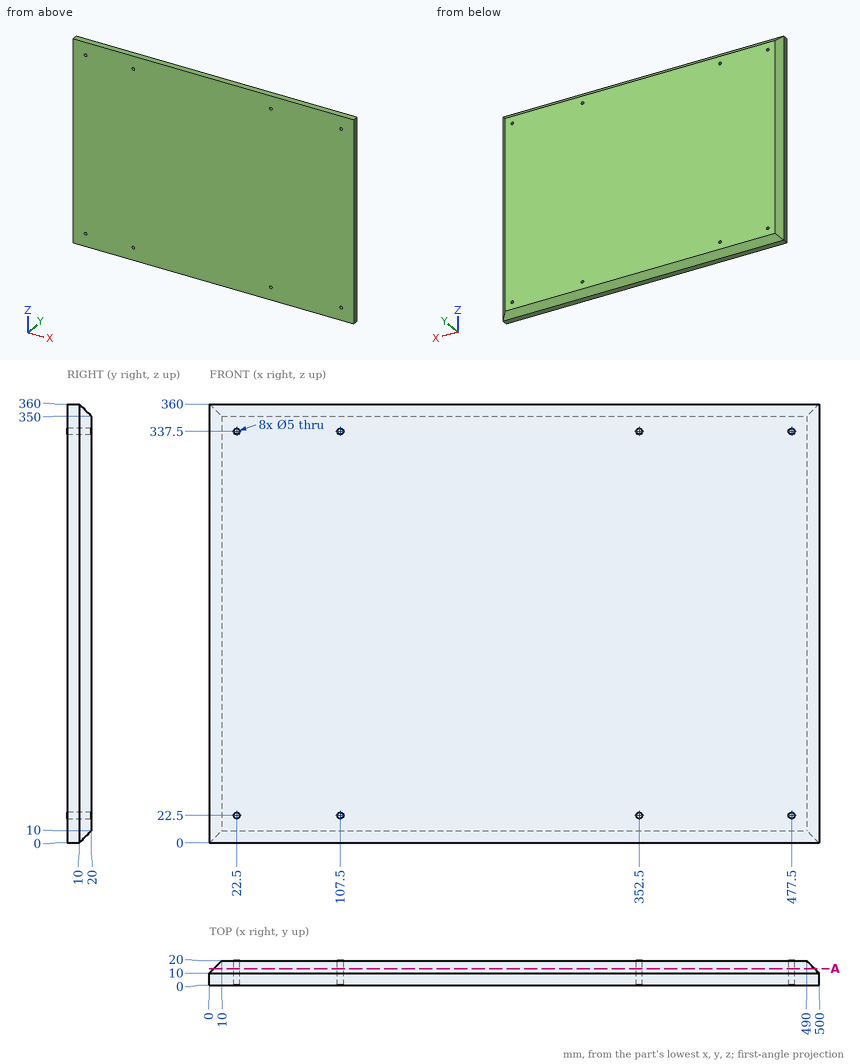
Verification items for this drawing (mm, ordinates from the low corner). Round coordinates to 2 decimals unless told otherwise and drop trailing zeros. Answer in a Markdown table with one row per item.
Q1. Go/stop test with flat-tipped pins: P1, Ø2, axis at x = 61.5, y = 15, coming from the -Z side; P2, Ø4, axis at y = 15.5, z = 283, coming from the -X side; P3, Ø4, axis at x = 52.5, y = 13, coming from the +Z side. Record where each tip stops, or that it passes through.
Data:
| item | result |
|---|---|
| P1 | stops at z = 4 |
| P2 | stops at x = 3.5 |
| P3 | stops at z = 359 |
Q2. Sectioned sample at A-A on y = 13.75. Give the number of separate pieces and of enclosed holes in the cut face, then the cut area to 3 significant figures.
Data:
| item | result |
|---|---|
| separate pieces | 1 |
| enclosed holes | 8 |
| area | 173,000 mm^2 |
Q3. Thickness scan on L1, parallel to X at y = 8.5, z = 337.5; L2, parallel to Z at x = 477.5, y = 6.75; L3, parallel to X at y = 16.75, z = 337. Record the ranges inside material, lowest first.
Data:
| item | result |
|---|---|
| L1 | x = 0 to 20, 25 to 105, 110 to 350, 355 to 475, 480 to 500 |
| L2 | z = 0 to 20, 25 to 335, 340 to 360 |
| L3 | x = 6.75 to 20.05, 24.95 to 105.05, 109.95 to 350.05, 354.95 to 475.05, 479.95 to 493.25 |
